from build123d import *

# Parameters (mm, degrees)
BOSS_EXTRUDE4_DEPTH = 5
SKETCH6_W           = 70
SKETCH6_H           = 70
BOSS_EXTRUDE5_DEPTH = 30
SKETCH8_R           = 3
CUT_EXTRUDE1_DEPTH  = 2
FILLET1_R           = 10
CUT_EXTRUDE2_DEPTH  = 30
BOSS_EXTRUDE6_DEPTH = 2.5
CHAMFER1_SIZE       = 1.25


with BuildPart() as part:
    # Sketch5 → Boss-Extrude4 (new body)
    with BuildSketch(Plane(origin=(0, 0, 0), x_dir=(1, 0, 0), z_dir=(0, 1, 0))):
        with BuildLine():
            Line((-22.5, -32.5), (22.5, -32.5))
            ThreePointArc((22.5, -32.5), (29.571067812, -29.571067812), (32.5, -22.5))
            Line((32.5, -22.5), (32.5, 22.5))
            ThreePointArc((32.5, 22.5), (29.571067812, 29.571067812), (22.5, 32.5))
            Line((22.5, 32.5), (-22.5, 32.5))
            ThreePointArc((-22.5, 32.5), (-29.571067812, 29.571067812), (-32.5, 22.5))
            Line((-32.5, 22.5), (-32.5, -22.5))
            ThreePointArc((-32.5, -22.5), (-29.571067812, -29.571067812), (-22.5, -32.5))
        make_face()
    extrude(amount=BOSS_EXTRUDE4_DEPTH)

    # Sketch6 → Boss-Extrude5 (add)
    with BuildSketch(Plane(origin=(0, 5, 0), x_dir=(1, 0, 0), z_dir=(0, 1, 0))):
        Rectangle(SKETCH6_W, SKETCH6_H)
    extrude(amount=BOSS_EXTRUDE5_DEPTH)

    # Sketch8 → Cut-Extrude1 (cut)
    with BuildSketch(Plane.XZ):
        with Locations(Location((26.037533906, -26.035533906, 0), (0, 0, 270))):
            Circle(SKETCH8_R)
        with Locations(Location((26.036533906, 26.036533906, 0), (0, 0, 270))):
            Circle(SKETCH8_R)
        with BuildLine():
            ThreePointArc((-23.035533906, 26.035533906), (-24.887483609, 28.807172503), (-28.156854249, 28.156854249))
            Line((-28.156854249, 28.156854249), (-23.914213562, 23.914213562))
            ThreePointArc((-23.914213562, 23.914213562), (-23.263895308, 24.887483609), (-23.035533906, 26.035533906))
        make_face()
        with BuildLine():
            Line((-23.914213562, 23.914213562), (-28.156854249, 28.156854249))
            ThreePointArc((-28.156854249, 28.156854249), (-28.156854249, 23.914213562), (-23.914213562, 23.914213562))
        make_face()
        with Locations(Location((-26.034533906, -26.036533906, 0), (0, 0, 270))):
            Circle(SKETCH8_R)
    extrude(amount=-CUT_EXTRUDE1_DEPTH, mode=Mode.SUBTRACT)

    # Fillet1
    fillet1_edges = [part.edges().sort_by_distance(p)[0] for p in [
        (-35, 20, -35),
        (-35, 20, 35),
        (35, 20, 35),
        (35, 20, -35),
    ]]
    fillet(fillet1_edges, radius=FILLET1_R)

    # Sketch9 → Cut-Extrude2 (cut)
    with BuildSketch(Plane(origin=(0, 35, 0), x_dir=(1, 0, 0), z_dir=(0, 1, 0))):
        with BuildLine():
            Line((25, 32.5), (-25, 32.5))
            ThreePointArc((-25, 32.5), (-30.303300859, 30.303300859), (-32.5, 25))
            Line((-32.5, 25), (-32.5, -25))
            ThreePointArc((-32.5, -25), (-30.303300859, -30.303300859), (-25, -32.5))
            Line((-25, -32.5), (25, -32.5))
            ThreePointArc((25, -32.5), (30.303300859, -30.303300859), (32.5, -25))
            Line((32.5, -25), (32.5, 25))
            ThreePointArc((32.5, 25), (30.303300859, 30.303300859), (25, 32.5))
        make_face()
    extrude(amount=-CUT_EXTRUDE2_DEPTH, mode=Mode.SUBTRACT)


with BuildPart() as cut_extrude2_piece_1:
    # of the separate pieces the step leaves, piece 1, a body of its own (cut_extrude2_pieces)
    add(part.part.solids().sort_by_distance((-22.5, 0, 32.5))[0])



with BuildPart() as cut_extrude2_piece_2:
    # of the separate pieces the step leaves, piece 2, a body of its own (cut_extrude2_pieces)
    add(part.part.solids().sort_by_distance((25, 5, -35))[0])


with BuildPart() as cut_extrude2_piece_1_1:
    add(cut_extrude2_piece_1.part)

    add(cut_extrude2_piece_2.part)  # Boss-Extrude6 merges Cut-Extrude2 piece 2
    # Sketch10 → Boss-Extrude6 (add)
    with BuildSketch(Plane.XZ.offset(-5)):
        with BuildLine():
            Line((-35, 25), (-35, -25))
            ThreePointArc((-35, -25), (-32.071067812, -32.071067812), (-25, -35))
            Line((-25, -35), (25, -35))
            ThreePointArc((25, -35), (32.071067812, -32.071067812), (35, -25))
            Line((35, -25), (35, 25))
            ThreePointArc((35, 25), (32.071067812, 32.071067812), (25, 35))
            Line((25, 35), (-25, 35))
            ThreePointArc((-25, 35), (-32.071067812, 32.071067812), (-35, 25))
        make_face()
    extrude(amount=-BOSS_EXTRUDE6_DEPTH)

    # Chamfer1
    chamfer1_edges = [cut_extrude2_piece_1_1.edges().sort_by_distance(p)[0] for p in [
        (0, 35, -32.5),
        (-30.303300859, 35, -30.303300859),
        (-32.5, 35, 0),
        (-30.303300859, 35, 30.303300859),
        (0, 35, 32.5),
        (30.303300859, 35, 30.303300859),
        (32.5, 35, 0),
        (30.303300859, 7.5, -30.303300859),
        (0, 7.5, -32.5),
        (-30.303300859, 7.5, -30.303300859),
        (-32.5, 7.5, 0),
        (-30.303300859, 7.5, 30.303300859),
        (0, 7.5, 32.5),
        (30.303300859, 7.5, 30.303300859),
        (32.5, 7.5, 0),
        (30.303300859, 35, -30.303300859),
    ]]
    chamfer(chamfer1_edges, length=CHAMFER1_SIZE)


solid = cut_extrude2_piece_1_1.part
Can you work these out from the model? Positions are in its coordinate system, mm. A direction names the side the tool comes from. Round coordinates to 2 decimals unless told otherwise and drop trailing zeros. Loops run counter-clockwise (first coordinate to the right, second up) from the corner with the lowest first, then second, coordinate; pieces in that order, holes last. Notation, with made-up numbers: (31, 10) - (36, 10) arc R31 ccw to (36, 45) - close; hole circle Ø8 at (52.5, -7). An arc over 180 degrees is marked (long way). Answer in a Markdown table with one row per item. Add a question column.
Q1. I want a section at B-B on x = 21.5. List the corners of the cut face in (y, z) for me.
Q2. Which directions (+Z, -Z, +X, -X, +Y, -Y) give clear straight access to the entire face, cutting with the end or side of a thin tool? Please do faces 4 (the flat face through (0, 2, 32.5)), 5 (the flat face through (-32.5, 21, 0)), 6 (the flat face through (26, 2, 26)), 7 (the cylindrical face through (29.65, 2.46, -29.49)).
Q3. I want a section at A-A on y = 16. List the corners of the cut face in (x, z) for me, and give its area (3 significant figures).
Q4. I want a section at C-C on z = 0. List the corners of the cut face in (x, y) for me, and give its area (4 significant figures).
Q5. I need wall thicknesses on L1, parallel to Z at x = 18.5, y = 32.5; L2, parallel to Y at x = 4, z = -9.5. Which ranges of each line are inside material? Lowest first, please.
Q6. For pin 1 Ø12 at (x, z) = (-18, 15.5) entering from +Y; pin 2 Ø5.5 at (y, z) = (1.5, -6.5) entering from +X; pin 3 Ø1.8 at (x, z) = (-25.5, -25.5) entering from -Y; pin 4 Ø6.5 at (x, z) = (26.5, 24.5) entering from -Y, each with a flat end and sliding along its axis, tell me the tip position at first contact or that it passes through.
Q7. We'd pull the mould along Z, two halves only. Please class faces 1 (the cylindrical face through (-30.361, 21.425, 30.245)), 2 (the flat face through (0, 20, -35)), 3 (the cylindrical face through (29.49, 2.46, 29.65)): pulls with the +Z half, pulls with the -Z half, needs draft (parallel to the pull), parting line crosses it, or undercut.
A:
| question | item | result |
|---|---|---|
| 1 | outline | (0, -32.5) - (5, -32.5) - (5, -35) - (35, -35) - (35, -33.75) - (33.75, -32.5) - (8.75, -32.5) - (7.5, -31.25) - (7.5, 31.25) - (8.75, 32.5) - (33.75, 32.5) - (35, 33.75) - (35, 35) - (5, 35) - (5, 32.5) - (0, 32.5) - close |
| 2 | face 4 | +Z, +X, -X, -Y |
| 2 | face 5 | +Y |
| 2 | face 6 | -Y |
| 2 | face 7 | -Z, +X, -Y |
| 3 | outline | (-35, -25) arc R10 ccw to (-25, -35) - (25, -35) arc R10 ccw to (35, -25) - (35, 25) arc R10 ccw to (25, 35) - (-25, 35) arc R10 ccw to (-35, 25) - close; hole (-32.5, -25) arc R7.5 ccw to (-25, -32.5) - (25, -32.5) arc R7.5 ccw to (32.5, -25) - (32.5, 25) arc R7.5 ccw to (25, 32.5) - (-25, 32.5) arc R7.5 ccw to (-32.5, 25) - close |
| 3 | area | 637 mm^2 |
| 4 | outline | (-35, 5) - (-32.5, 5) - (-32.5, 0) - (32.5, 0) - (32.5, 5) - (35, 5) - (35, 35) - (33.75, 35) - (32.5, 33.75) - (32.5, 8.75) - (31.25, 7.5) - (-31.25, 7.5) - (-32.5, 8.75) - (-32.5, 33.75) - (-33.75, 35) - (-35, 35) - close |
| 4 | area | 637.5 mm^2 |
| 5 | L1 | -35 to -32.5, 32.5 to 35 |
| 5 | L2 | 0 to 7.5 |
| 6 | pin 1 | y = 7.5 |
| 6 | pin 2 | x = 32.5 |
| 6 | pin 3 | y = 2 |
| 6 | pin 4 | y = 0 |
| 7 | face 1 | undercut |
| 7 | face 2 | pulls with the -Z half |
| 7 | face 3 | pulls with the +Z half |
